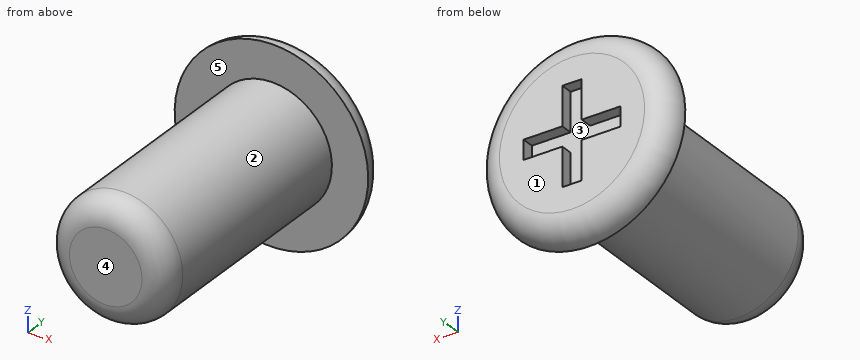
from build123d import *

# Parameters (mm, degrees)
SKETCH1_R           = 6.35
BOSS_EXTRUDE1_DEPTH = 25.4
SKETCH2_R           = 10.16
BOSS_EXTRUDE2_DEPTH = 2.54
FILLET1_R           = 2.54
SKETCH3_W           = 4.064
SKETCH3_H           = 2.032
SKETCH3_W_2         = 2.032
SKETCH3_H_2         = 4.064
CUT_EXTRUDE1_DEPTH  = 1.27
FILLET2_R           = 2.54


with BuildPart() as part:
    # Sketch1 → Boss-Extrude1 (new body)
    with BuildSketch(Plane(origin=(0, 0, 0), x_dir=(1, 0, 0), z_dir=(0, 1, 0))):
        with Locations(Location((0, 0, 0), (0, 0, 270))):
            Circle(SKETCH1_R)
    extrude(amount=BOSS_EXTRUDE1_DEPTH)

    # Sketch2 → Boss-Extrude2 (add)
    with BuildSketch(Plane(origin=(0, 25.4, 0), x_dir=(1, 0, 0), z_dir=(0, 1, 0))):
        with Locations(Location((0, 0, 0), (0, 0, 270))):
            Circle(SKETCH2_R)
    extrude(amount=BOSS_EXTRUDE2_DEPTH)

    # Fillet1
    fillet1_edges = [part.edges().sort_by_distance(p)[0] for p in [
        (0, 27.94, -10.16),
    ]]
    fillet(fillet1_edges, radius=FILLET1_R - 0.0001)  # a hair under: the kernel refuses the full size

    # Sketch3 → Cut-Extrude1 (cut)
    with BuildSketch(Plane(origin=(0, 27.94, 0), x_dir=(1, 0, 0), z_dir=(0, 1, 0))):
        with Locations((-3.048, 0)):
            Rectangle(SKETCH3_W, SKETCH3_H)
        with Locations((0, 3.048)):
            Rectangle(SKETCH3_W_2, SKETCH3_H_2)
        with Locations((3.048, 0)):
            Rectangle(SKETCH3_W, SKETCH3_H)
        Rectangle(SKETCH3_W_2, SKETCH3_H)
        with Locations((0, -3.048)):
            Rectangle(SKETCH3_W_2, SKETCH3_H_2)
    extrude(amount=-CUT_EXTRUDE1_DEPTH, mode=Mode.SUBTRACT)

    # Fillet2
    fillet2_edges = [part.edges().sort_by_distance(p)[0] for p in [
        (0, 0, -6.35),
    ]]
    fillet(fillet2_edges, radius=FILLET2_R)


solid = part.part
For this review, take the finished solid that the model builds, in its own axes (mm). Face numbers are marked on the shaded views. A direction names the side the tool comes from. Round coordinates to 2 decimals unless told otherwise and drop trailing zeros. Loops run counter-clockwise (first coordinate to the right, second up) from the corner with the lowest first, then second, coordinate; pieces in that order, holes last. Notation, with made-up numbers: (25, 69.5) - (64, 69.5) arc R20 cw to (64, 97.5) - close; hole circle Ø7 at (54.25, 12). An arc over 180 degrees is marked (long way). Use one line per item in the form item = value.
Item 1: For line 1 (Y direction, x = 6.5, z = 0.75); line 2 (Y direction, x = 4, z = 8); line 3 (X direction, y = 12, z = 1), list the stretches that pass through material, from the lowest coordinate up.
Answers:
line_1 = 25.4 to 27.94
line_2 = 25.4 to 27.57
line_3 = -6.27 to 6.27
Item 2: Mouldability with a two-part tool opening along Z and no side actions: class the marked faces 1, 2 and 3 as +Z half, -Z half, draft (parallel to the pull), parting line (faces both ways), or undercut.
Answers:
face_1 = draft
face_2 = parting line
face_3 = undercut
Item 3: Consider section D-D on y = 2. Write out the cut boundary in (x, z), then the cut area to 3 significant figures.
Answers:
outline = circle Ø12.58 at (0, 0)
area = 124 mm^2
Item 4: Clearance check with flat-ended pins moving along their axes: P1, Ø6, axis at x = 5, y = 3, coming from the +Z side; P2, Ø1.4, axis at y = 27, z = -3, coming from the +X side; P3, Ø1, axis at y = 27.5, z = 0, coming from the -X side. State where each tip first meets the part, or that it passes through.
Answers:
P1 = 6.03
P2 = 9.6
P3 = -9.59
Item 5: Consider section C-C on y = 6.5. Write out the cut boundary in (x, z), then the cut area to 3 significant figures.
Answers:
outline = circle Ø12.7 at (0, 0)
area = 127 mm^2
Item 6: Tool access review of the marked faces 4 and 5: name each direction out of +Z, -Z, +X, -X, +Y, -Y from which nothing blocks a thin tool from reaching the whole face with its end or side.
Answers:
face_4 = +Z, -Z, +X, -X, -Y
face_5 = -Y
